Work out the finished part from the listing and answer in its coordinate system (mm). A direction names the side the tool comes from. Give positions to 0.01 mm unless a question says otherwise; leave off trailing zeros. Loops run counter-clockwise (first coordinate to the right, second up) from the corner with the lowest first, then second, coordinate; pieces in that order, holes last. Notation, with made-up numbers: M -1.5,48.25 L 31.5,48.25 A12 cw 31.5,58.25 Z; hole C 36,-5.5 d3. An arc over 180 degrees is marked long. Use a Markdown table: item, result.
```python
from build123d import *

# Parameters (mm, degrees)
SKETCH1_W           = 97
SKETCH1_H           = 200
BOSS_EXTRUDE1_DEPTH = 42
SKETCH3_R           = 1.5
CUT_EXTRUDE1_DEPTH  = 3
SKETCH4_W           = 97
SKETCH4_H           = 200
SKETCH4_W_2         = 89.324278463
SKETCH4_H_2         = 130.340528777
CUT_EXTRUDE2_DEPTH  = 227.214499977
SKETCH5_W           = 71.136204213
SKETCH5_H           = 114.608329011
CUT_EXTRUDE3_DEPTH  = 213.410706636
SKETCH6_W           = 89.324278463
SKETCH6_H           = 39
CUT_EXTRUDE4_DEPTH  = 166.700724789


with BuildPart() as part:
    # Sketch1 → Boss-Extrude1 (new body)
    with BuildSketch(Plane(origin=(0, 0, 0), x_dir=(1, 0, 0), z_dir=(0, 1, 0))):
        with Locations((48.5, 100)):
            Rectangle(SKETCH1_W, SKETCH1_H)
    extrude(amount=BOSS_EXTRUDE1_DEPTH)

    # Sketch3 → Cut-Extrude1 (cut)
    with BuildSketch(Plane(origin=(0, 42, 0), x_dir=(1, 0, 0), z_dir=(0, 1, 0))):
        with Locations(Location((88.5, 61, 0), (0, 0, 270))):
            Circle(SKETCH3_R)
        with Locations(Location((8.5, 61, 0), (0, 0, 270))):
            Circle(SKETCH3_R)
        with Locations(Location((88.5, 181, 0), (0, 0, 270))):
            Circle(SKETCH3_R)
        with Locations(Location((8.5, 181, 0), (0, 0, 270))):
            Circle(SKETCH3_R)
    extrude(amount=-CUT_EXTRUDE1_DEPTH, mode=Mode.SUBTRACT)

    # Sketch4 → Cut-Extrude2 (cut, through all)
    with BuildSketch(Plane(origin=(0, 42, 0), x_dir=(1, 0, 0), z_dir=(0, 1, 0))):
        with Locations((48.5, 100)):
            Rectangle(SKETCH4_W, SKETCH4_H)
        with Locations((48.633502434, 120.975462234)):
            Rectangle(SKETCH4_W_2, SKETCH4_H_2, mode=Mode.SUBTRACT)
    extrude(amount=-CUT_EXTRUDE2_DEPTH, mode=Mode.SUBTRACT)

    # Sketch5 → Cut-Extrude3 (cut, through all)
    with BuildSketch(Plane(origin=(0, 42, 0), x_dir=(1, 0, 0), z_dir=(0, 1, 0))):
        with Locations((48.992776193, 120.706006915)):
            Rectangle(SKETCH5_W, SKETCH5_H)
    extrude(amount=-CUT_EXTRUDE3_DEPTH, mode=Mode.SUBTRACT)

    # Sketch6 → Cut-Extrude4 (cut, through all)
    with BuildSketch(Plane(origin=(0, 0, -186.145726622), x_dir=(-1, 0, 0), z_dir=(0, 0, -1))):
        with Locations((-48.633502434, 19.5)):
            Rectangle(SKETCH6_W, SKETCH6_H)
    extrude(amount=-CUT_EXTRUDE4_DEPTH, mode=Mode.SUBTRACT)


solid = part.part
```
(1) A cutting plane is placed at C-C (y = 41.1). Write down the section's boundary in (x, z).
Entries:
| item | result |
|---|---|
| outline | M 3.97,-186.15 L 93.3,-186.15 L 93.3,-55.81 L 3.97,-55.81 Z; hole C 8.5,-181 d3; hole C 8.5,-61 d3; hole M 13.42,-178.01 L 84.56,-178.01 L 84.56,-63.4 L 13.42,-63.4 Z; hole C 88.5,-181 d3; hole C 88.5,-61 d3 |
(2) A cutting plane is placed at A-A (z = -119.5). Write down the section's boundary in (x, y).
Entries:
| item | result |
|---|---|
| outline | M 3.97,39 L 13.42,39 L 13.42,42 L 3.97,42 Z; M 84.56,39 L 93.3,39 L 93.3,42 L 84.56,42 Z |
(3) Consider probe 1 along X at (y, z) = (41.1, -181); probe 2 along Z at (x, y) = (88.5, 39.95); probe 3 along X at (y, z) = (41.1, -148.5). Determine where each line is inside the solid, lowest interval first. Write a range as [from, to].
Entries:
| item | result |
|---|---|
| probe 1 | x = [3.97, 7], [10, 87], [90, 93.3] |
| probe 2 | z = [-186.15, -182.5], [-179.5, -62.5], [-59.5, -55.81] |
| probe 3 | x = [3.97, 13.42], [84.56, 93.3] |
(4) The mould has two halves that part along Z. Classify faces 1 (the flat face through (93.296, 41, -120)), 2 (the flat face through (48, 41, -186.146)), 3 (the flat face through (13.425, 41, -120)): released by +Z, released by -Z, zero draft, split by the parting line, or undercut.
Entries:
| item | result |
|---|---|
| face 1 | zero draft |
| face 2 | released by -Z |
| face 3 | undercut |
(5) A cutting plane is placed at D-D (z = -61). Write down the section's boundary in (x, y), and give its area (3 significant figures).
Entries:
| item | result |
|---|---|
| outline | M 3.97,39 L 7,39 L 7,42 L 3.97,42 Z; M 10,39 L 87,39 L 87,42 L 10,42 Z; M 90,39 L 93.3,39 L 93.3,42 L 90,42 Z |
| area | 250 mm² |
(6) Which of the six approach directions +Z, -Z, +X, -X, +Y, -Y give full straight-line access (tool end or side, diameter ignored) to faces 4 (the flat face through (48, 41, -55.805)), 5 (the flat face through (48, 41, -178.01))?
Entries:
| item | result |
|---|---|
| face 4 | +Z, +X, -X, +Y, -Y |
| face 5 | +Y, -Y |
(7) A cutting plane is placed at B-B (x = 88.5). Write down the section's boundary in (y, z).
Entries:
| item | result |
|---|---|
| outline | M 39,-186.15 L 42,-186.15 L 42,-182.5 L 39,-182.5 Z; M 39,-179.5 L 42,-179.5 L 42,-62.5 L 39,-62.5 Z; M 39,-59.5 L 42,-59.5 L 42,-55.81 L 39,-55.81 Z |
